```python
from build123d import *
from build123d.topology import SkipClean

# Parameters (mm, degrees)
SKETCH1_R                = 5.75
SKETCH1_R_2              = 3
BOSS_EXTRUDE1_DEPTH      = 1.5
SKETCH2_R                = 5
BOSS_EXTRUDE2_DEPTH      = 16
BOSS_EXTRUDE2_TAPER      = 1
FILLET1_R                = 1
BOSS_EXTRUDE3_REACH      = 22.208
BOSS_EXTRUDE3_END_RADIUS = 5.75
SKETCH4_W                = 1
SKETCH4_H                = 16.9
FILLET2_R                = 2
CUT_EXTRUDE1_DEPTH       = 10
BOSS_EXTRUDE4_START      = 5.75
SKETCH6_W                = 1
SKETCH6_H                = 6
BOSS_EXTRUDE4_DEPTH      = 0.5


# Read off the part's stored shape, not the designer's step: Dome1
with BuildPart() as part:
    # Sketch1 → Boss-Extrude1 (new body)
    with BuildSketch(Plane(origin=(0, 0, 0), x_dir=(1, 0, 0), z_dir=(0, 1, 0))):
        with Locations(Location((0, 0, 0), (0, 0, 270))):
            Circle(SKETCH1_R)
        with Locations(Location((0, 0, 0), (0, 0, 270))):
            Circle(SKETCH1_R_2, mode=Mode.SUBTRACT)
    extrude(amount=BOSS_EXTRUDE1_DEPTH)

    # Sketch2 → Boss-Extrude2 (add)
    with BuildSketch(Plane(origin=(0, 1.5, 0), x_dir=(1, 0, 0), z_dir=(0, 1, 0))):
        Circle(SKETCH2_R)
    extrude(amount=BOSS_EXTRUDE2_DEPTH, taper=BOSS_EXTRUDE2_TAPER)

    # Dome1 outline → Dome1 (revolve)
    with BuildSketch(Plane.XY):
        with BuildLine():
            Line((0, 17.5), (4.720718972, 17.499999995))
            ThreePointArc((4.720718972, 17.499999995), (2.412736394, 18.247256658), (0, 18.5))
            Line((0, 18.5), (0, 17.5))
        make_face()
    revolve(axis=Axis((0, 0, 0), (0, 1, 0)))

    # Fillet1
    fillet1_edges = [part.edges().sort_by_distance(p)[0] for p in [
        (-4.720718961, 17.5, 0),
    ]]
    fillet(fillet1_edges, radius=FILLET1_R)

    # Boss-Extrude3: up to this cylinder (the profile starts inside it)
    with SkipClean():  # the faces are left unmerged after this step: merging them gives an invalid solid
        boss_extrude3_end = Plane(origin=(0, 9.95, 0), z_dir=(0, -1, 0)) * Cylinder(BOSS_EXTRUDE3_END_RADIUS, 56.916, mode=Mode.PRIVATE)
        # Sketch4 → Boss-Extrude3 (add, up to the surface)
        with BuildSketch(Plane(origin=(0, 0, 0), x_dir=(0, 0, -1), z_dir=(1, 0, 0)), mode=Mode.PRIVATE) as boss_extrude3_sk1:
            with Locations((0, 9.95)):
                Rectangle(SKETCH4_W, SKETCH4_H)
        boss_extrude3_tool1 = extrude(boss_extrude3_sk1.sketch, amount=BOSS_EXTRUDE3_REACH, mode=Mode.PRIVATE) & boss_extrude3_end
        add(boss_extrude3_tool1.solids().sort_by_distance((0, 9.95, 0))[0])

    # Fillet2
    fillet2_edges = [part.edges().sort_by_distance(p)[0] for p in [
        (5.75, 18.4, 0),
    ]]
    fillet(fillet2_edges, radius=FILLET2_R)

    # Sketch5 → Cut-Extrude1 (cut)
    with BuildSketch(Plane(origin=(0, 0, 0), x_dir=(1, 0, 0), z_dir=(0, 1, 0))):
        with BuildLine():
            Line((-2.236067977, 2), (2.236067977, 2))
            ThreePointArc((2.236067977, 2), (0, -3), (-2.236067977, 2))
        make_face()
    extrude(amount=CUT_EXTRUDE1_DEPTH, mode=Mode.SUBTRACT)

    # Sketch6 → Boss-Extrude4 (add)
    with BuildSketch(Plane(origin=(0, 0, 0), x_dir=(0, 0, -1), z_dir=(1, 0, 0)).offset(BOSS_EXTRUDE4_START)):
        with Locations((0, 3)):
            Rectangle(SKETCH6_W, SKETCH6_H)
    extrude(amount=-BOSS_EXTRUDE4_DEPTH)


solid = part.part
```
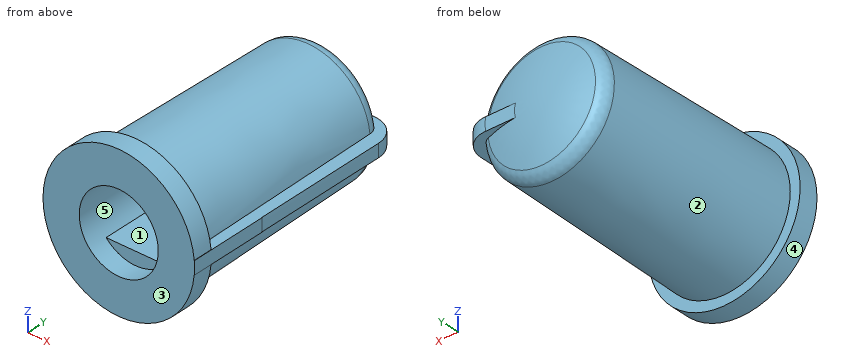
Geometry check sheet. Reference: the model listing, model coordinates, mm. Face numbers are marked on the shaded views. A direction names the side the tool comes from. Coordinates: 2 decimals unless noted, no trailing zeros. Order: outer loops, then holes, each group sorted by start corner. A loop starts at its lowest first (then second) coordinate and runs counter-clockwise, first axis right, second up. Notation, with made-up numbers: (6.5, -23.75) - (45.5, -23.75) arc R14 cw to (45.5, -2.75) - close; hole circle Ø2 at (16, 41.25). An arc over 180 degrees is marked (long way). Answer as a JSON object with one key per item and string values. Group by question number.
Item 1: Depth check by flat-ended pin: pin 1 Ø1 at (y, z) = (5.5, -1.5) entering from -X; pin 2 Ø1.3 at (x, y) = (4.5, 12) entering from -Z; pin 3 Ø0.8 at (x, z) = (2.5, 0) entering from +Y. Enter the tip coordinate at first touch or a pass-through.
Item 2: Scan lines: probe 1 along Z at (x, y) = (5, 7.75); probe 2 along Z at (x, y) = (0, 6.5); probe 3 along X at (y, z) = (9, 0.25). Record each from-to range of solid material in increasing order.
Item 3: Tool access check on the marked faces 4 and 5. Record the directions out of +Z, -Z, +X, -X, +Y, -Y that give a thin tool (end or side, any length) a straight path to the whole face; none if there is none.
Item 4: Sectioned sample at C-C, the plane y = 14. Record the cut outline in (x, z).
Item 5: Sectioned sample at A-A, the plane y = 8.5. Record the cut outline in (x, z), and give its area (3 significant figures).
Item 6: Sectioned sample at B-B, the plane y = 6.25. Record the cut outline in (x, z).
Item 7: Draft check along X on the marked faces 1, 2 and 3. Enter one of: +X half, -X half, draft (parallel to the pull), parting line (faces both ways), or undercut.
Resolved:
{
 "1": {"pin 1": "x = -4.83", "pin 2": "z = -2.89", "pin 3": "y = 18.4"},
 "2": {"probe 1": "-0.5 to 0.5", "probe 2": "-4.91 to -2, 3 to 4.91", "probe 3": "-4.86 to -2.99, 2.99 to 5.74"},
 "3": {"face 4": "+Y, -Y", "face 5": "-Y"},
 "4": {"outline": "(4.76, -0.5) - (5.73, -0.5) arc R5.75 ccw to (5.73, 0.5) - (4.76, 0.5) arc R4.78 ccw (long way) to start"},
 "5": {"outline": "(4.85, -0.5) - (5.73, -0.5) arc R5.75 ccw to (5.73, 0.5) - (4.85, 0.5) arc R4.88 ccw (long way) to start; hole (-2.24, -2) - (2.24, -2) arc R3 ccw (long way) to start", "area": "50.4 mm^2"},
 "6": {"outline": "(4.89, -0.5) - (5.73, -0.5) arc R5.75 ccw to (5.73, 0.5) - (4.89, 0.5) arc R4.92 ccw (long way) to start; hole (-2.24, -2) - (2.24, -2) arc R3 ccw (long way) to start"},
 "7": {"face 1": "undercut", "face 2": "parting line", "face 3": "draft"}
}
